from build123d import *

# Parameters (mm, degrees)
F0_R          = 25.4
F0_R_2        = 19.05
F1_DEPTH      = 25.4
F1_DEPTH_BACK = 25.4
F2_W          = 30.48
F2_H          = 11.43
F2_W_2        = 25.4
F2_H_2        = 6.35
F3_DEPTH      = 127
F4_DEPTH      = 25.401
F4_DEPTH_BACK = 25.401


with BuildPart() as f1:
    # F0 (on Top) → F1 (new body, two sides)
    with BuildSketch(Plane.XY) as f1_sk:
        Circle(F0_R)
        Circle(F0_R_2, mode=Mode.SUBTRACT)
    extrude(amount=F1_DEPTH)
    extrude(f1_sk.sketch, amount=-F1_DEPTH_BACK)

    # F2 (on Front) → F3 (join)
    with BuildSketch(Plane.XZ):
        Rectangle(F2_W, F2_H)
        Rectangle(F2_W_2, F2_H_2, mode=Mode.SUBTRACT)
    extrude(amount=F3_DEPTH)

    # F0 (on Top) → F4 (cut, two sides)
    with BuildSketch(Plane.XY) as f4_sk:
        Circle(F0_R_2)
    extrude(amount=-F4_DEPTH, mode=Mode.SUBTRACT)
    extrude(f4_sk.sketch, amount=F4_DEPTH_BACK, mode=Mode.SUBTRACT)


solid = f1.part
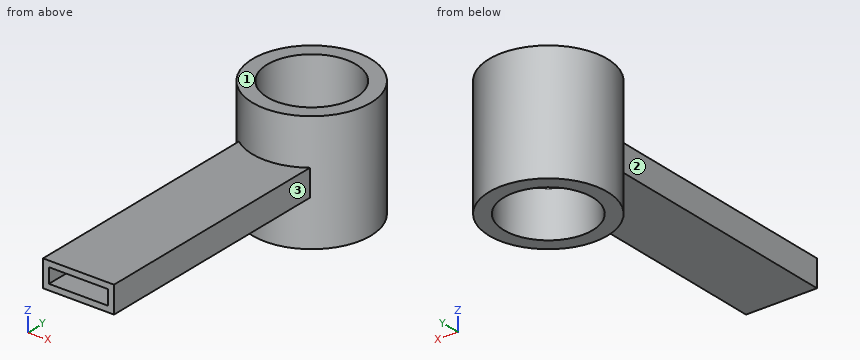
For this review, take the finished solid that the model builds, in its own axes (mm). Face numbers are marked on the shaded views. A direction names the side the tool comes from. Give positions to 0.01 mm unless a question says otherwise; leave off trailing zeros. Loops run counter-clockwise (first coordinate to the right, second up) from the corner with the lowest first, then second, coordinate; pieces in that order, holes last. Notation, with made-up numbers: M 40.25,62 L 91.25,62 A16 ccw 91.25,76 Z; hole C 56,-16.75 d10. An arc over 180 degrees is marked long. Put each result on its own line as item: value. Start each with the question number.
(1) Add section B-B, the plane x = 5. Write out the cut boundary in (y, z) (3 decimals).
(2) Add section D-D, the plane z = -19.5. Write out the cut boundary in (x, y), then the cut area to 3 significant figures.
(3) Add section C-C, the plane y = 0. Write out the cut boundary in (x, z).
(4) Wall thickness on L1, parallel to Z at x = 3, y = -113 (3 decimals); L2, parallel to Y at x = 0, z = -17; L3, parallel to X at y = -107, z = 2.5: over which ranges is each line inside the solid? List them lowest first.
(5) For pin 1 (9 mm diameter, centred on y = -75, z = -1, fed in from +X); pin 2 (3 mm diameter, centred on y = -81, z = -1.5, fed in from -X); pin 3 (1 mm diameter, centred on x = 15.5, y = -61, fed in from -Z) (3 decimals), all flat-tipped, find the tip position at first contact; note any pin that passes through.
(6) Add section A-A, the plane y = -43.5. Write out the cut boundary in (x, z) (3 decimals).
(7) Machinability: for the marked faces 1, 2 and 3, which of the approach directions +Z, -Z, +X, -X, +Y, -Y give a long, thin tool a straight path to every point of the face, cutting with its end or side? Answer none if there is none.
Result:
1. outline: M -127,-5.715 L -24.903,-5.715 L -24.903,-25.4 L -18.382,-25.4 L -18.382,25.4 L -24.903,25.4 L -24.903,5.715 L -127,5.715 L -127,3.175 L -24.903,3.175 L -24.903,-3.175 L -127,-3.175 Z; M 18.382,-25.4 L 24.903,-25.4 L 24.903,25.4 L 18.382,25.4 Z
2. outline: C 0,0 d50.8; hole C 0,0 d38.1
2. area: 887 mm^2
3. outline: M -25.4,-25.4 L -19.05,-25.4 L -19.05,25.4 L -25.4,25.4 Z; M 19.05,-25.4 L 25.4,-25.4 L 25.4,25.4 L 19.05,25.4 Z
4. L1: z = -5.715 to -3.175, 3.175 to 5.715
4. L2: y = -25.4 to -19.05, 19.05 to 25.4
4. L3: x = -15.24 to -12.7, 12.7 to 15.24
5. pin 1: stops at x = 15.24
5. pin 2: stops at x = -15.24
5. pin 3: stops at z = -5.715
6. outline: M -15.24,-5.715 L 15.24,-5.715 L 15.24,5.715 L -15.24,5.715 Z; hole M -12.7,-3.175 L 12.7,-3.175 L 12.7,3.175 L -12.7,3.175 Z
7. face 1: +Z, +X, -X, +Y, -Y
7. face 2: +Z, -Z, -X, -Y
7. face 3: +Z, -Z, +X, -Y
